Work out the finished part from the listing and answer in its coordinate system (mm). A direction names the side the tool comes from. Coordinates: 2 decimals unless noted, no trailing zeros. Order: outer loops, then holes, each group sorted by start corner. A loop starts at its lowest first (then second) coordinate and runs counter-clockwise, first axis right, second up. Notation, with made-up numbers: M 71,-10.5 L 89,-10.5 A12 ccw 89,4.5 Z; hole C -16.75,74 d6. An arc over 180 degrees is marked long. Write item = value, one per line. Start each with the question number.
Q1. A tool of negligible diameter and unlimited length cuts with its end or side. For faces 1 (the flat face through (0.5, 0.5, 7.5)), 2 (the flat face through (0, 0, 0)), from which of +Z, -Z, +X, -X, +Y, -Y can it reach the whole face along a straight path? Write none if from no direction.
Q2. Find section B-B on x = 0. Give the vertices of the cut face in (y, z), and give its area (3 significant figures).
Q3. Find section A-A on y = 0.45. Give the vertices of the cut face in (x, z), and give its area (3 significant figures).
Q4. Straight lines are drawn through the part: line 1 along X through (y, z) = (0.55, 0.25); line 2 along X through (y, z) = (0.3, 6.25); line 3 along Z through (x, y) = (-7.5, 0.65). For each, find the intervals that lie inside material, in ascending order.
Q5. Determine the mould class of faces 3 (the flat face through (0, 1, 0)), 4 (the cylindrical face through (-0.01, 0.49, 5.75)), 5 (the flat face through (-0.5, 0.5, 7.5)) for opening direction X: released by +X, released by -X, zero draft, split by the parting line, or undercut.
Q6. Find section C-C on z = -7. Give the vertices of the cut face in (x, y), and give its area (3 significant figures).
Q7. This flat-tipped pin is pushed along its axis until it touches: P1, Ø0.5, axis at y = 0.5, z = 8, coming from the +X side. Where does it stop, or does it pass through?
```python
from build123d import *

# Parameters (mm, degrees)
BOSS_EXTRUDE1_DEPTH = 1


with BuildPart() as part:
    # Sketch1 → Boss-Extrude1 (new body)
    with BuildSketch(Plane(origin=(0, 0, 0), x_dir=(1, 0, 0), z_dir=(0, 1, 0))):
        with BuildLine():
            ThreePointArc((8.75, 0), (-6.00780742, 6.361505325), (-0.5, -8.735702605))
            Line((-0.5, -8.735702605), (-0.5, -6.25))
            ThreePointArc((-0.5, -6.25), (0, -5.75), (0.5, -6.25))
            Line((0.5, -6.25), (0.5, -8.735702605))
            ThreePointArc((0.5, -8.735702605), (6.361505325, -6.00780742), (8.75, 0))
        make_face()
    extrude(amount=BOSS_EXTRUDE1_DEPTH)


solid = part.part
```
Findings below:
q1.face_1 = +Z, +Y, -Y
q1.face_2 = +Z, -Z, +X, -X, -Y
q2.outline = M 0,-8.75 L 1,-8.75 L 1,5.75 L 0,5.75 Z
q2.area = 14.5 mm^2
q3.outline = M -0.5,6.25 L -0.5,8.74 A8.75 ccw long 0.5,8.74 L 0.5,6.25 A0.5 cw Z
q3.area = 238 mm^2
q4.line_1 = -8.75 to 8.75
q4.line_2 = -6.12 to -0.5, 0.5 to 6.12
q4.line_3 = -4.51 to 4.51
q5.face_3 = zero draft
q5.face_4 = undercut
q5.face_5 = undercut
q6.outline = M -5.25,0 L 5.25,0 L 5.25,1 L -5.25,1 Z
q6.area = 10.5 mm^2
q7.P1 = 4.06
